Autodesk Inventor part; units mm, degrees
ref_plane "YZ Plane" through (0, 0, 0) normal (1, 0, 0) x (0, 1, 0)
ref_plane "XZ Plane" through (0, 0, 0) normal (0, 1, 0) x (-1, 0, 0)
ref_plane "XY Plane" through (0, 0, 0) normal (0, 0, 1) x (1, 0, 0)
sketch "Sketch1" plane through (0, 0, 0) normal (0, 1, 0) x (-1, 0, 0)
  line L0 (-31, -16.75) -> (31, -16.75)
  line L1 (31, -16.75) -> (31, 16.75)
  line L2 (31, 16.75) -> (-31, 16.75)
  line L3 (-31, 16.75) -> (-31, -16.75)
  line L4 (-31, -16.75) -> (31, 16.75) construction
  line L5 (31, -16.75) -> (-31, 16.75) construction
  point P0 (0, 0)
  dimension "d0" = 33.5
  dimension "d1" = 62
extrude "Extrusion1" add sketch "Sketch1" along normal blind 1.5
fillet "Fillet1" radius 2 4 edges at (31, 0.75, 16.75) (31, 0.75, -16.75) (-31, 0.75, -16.75) (-31, 0.75, 16.75)
sketch "Sketch5" plane through (0, 0, 0) normal (0, -1, 0) x (1, 0, 0)
  line L0 (41, -5) -> (31, -5)
  line L1 (31, -5) -> (31, 5)
  line L2 (31, 5) -> (41, 5)
  line L3 (41, 5) -> (41, -5)
  line L4 (41, -5) -> (31, 5) construction
  line L5 (31, -5) -> (41, 5) construction
  line L6 (31, 14.75) -> (31, -14.75)
  line L7 (-41, -5) -> (-31, -5)
  line L8 (-31, -5) -> (-31, 5)
  line L9 (-31, 5) -> (-41, 5)
  line L10 (-41, 5) -> (-41, -5)
  line L11 (-41, -5) -> (-31, 5) construction
  line L12 (-31, -5) -> (-41, 5) construction
  line L13 (-31, -14.75) -> (-31, 14.75)
  point P0 (0, 0)
  point P1 (36, 0)
  point P2 (36, 0)
  point P3 (-36, 0)
  point P4 (-36, 0)
  dimension "d37" = 10
  dimension "d38" = 10
extrude "Extrusion6" add sketch "Sketch5" against normal up to surface (1.5 mm away)
sketch "Sketch6" plane through (0, 0, 0) normal (0, -1, 0) x (1, 0, 0)
  circle A0 centre (36, 0) radius 1.75
  line L0 (31, 14.75) -> (31, 5)
  circle A1 centre (-36, 0) radius 1.75
  line L1 (-31, 5) -> (-31, 14.75)
  point P0 (0, 0)
  dimension "d41" = 3.5
  dimension "d42" = 5
  dimension "d51" = 5
extrude "Extrusion7" cut sketch "Sketch6" against normal up to surface (1.5 mm away)
fillet "Fillet6" radius 2 8 edges at (31, 0.75, 5) (41, 0.75, 5) (41, 0.75, -5) (31, 0.75, -5) (-31, 0.75, 5) (-41, 0.75, 5) (-41, 0.75, -5) (-31, 0.75, -5)
chamfer "Chamfer1" distance 1.5 angle 45 2 edges at (34.25, 0, 0) (-37.75, 0, 0)
equation "\"d51\" = d42"
properties part number "BatteryPlate"
The listing builds one solid part. Answer for the finished solid, in the listing's coordinates (mm). A direction names the side the tool comes from. Give positions to 0.01 mm unless a question says otherwise; leave off trailing zeros. Order: outer loops, then holes, each group sorted by start corner. A loop starts at its lowest first (then second) coordinate and runs counter-clockwise, first axis right, second up. Notation, with made-up numbers: (70.5, -2) -> (83.5, -2) arc R24 ccw to (83.5, 14) -> close; hole circle Ø5 at (51.25, -36). An arc over 180 degrees is marked (long way). Answer as a JSON object with one key per item and string values. Group by question number.
Item 1: The part is cut by section C-C on y = 0.7. Write down the section's boundary in (x, z), and give its area (3 significant figures).
Item 2: A tool of negligible diameter and unlimited length cuts with its end or side. For faces 1 (the flat face through (36, 1, 5)), 2 (the flat face through (-36, 1, 5)), 3 (the flat face through (36, 1, -5)), 4 (the flat face through (0, 1, -16.75)), 5 (the flat face through (-36, 1, -5)), from which of +Z, -Z, +X, -X, +Y, -Y can it reach the whole face along a straight path? Write none if from no direction.
Item 3: Flat-ended cylindrical pins translate along their axes: pin 1 (0.8 mm diameter, centred on y = 1, z = -11.5, fed in from -X); pin 2 (0.8 mm diameter, centred on x = 36, y = 1, fed in from -Z); pin 3 (0.8 mm diameter, centred on x = -36, y = 0.5, fed in from +Z). Find the tip coordinate at first contact, or state that the pin passes through.
Item 4: The part is cut by section D-D on z = -11.5. Write down the section's boundary in (x, y).
Item 5: The part is cut by section A-A on z = 0. Give the number of separate pieces and of enclosed holes in the cut face, and give its area (3 significant figures).
Item 6: Consider L1, parallel to X at y = 0.75, z = -0.5; L2, parallel to X at y = 0.7, z = -1; L3, parallel to X at y = 0.7, z = 13. Determine where each line is inside the solid, lowest interval first. Write a range as from..to.
Result set:
{
 "1": {"outline": "(-41, -3) arc R2 ccw to (-39, -5) -> (-33, -5) arc R2 cw to (-31, -7) -> (-31, -14.75) arc R2 ccw to (-29, -16.75) -> (29, -16.75) arc R2 ccw to (31, -14.75) -> (31, -7) arc R2 cw to (33, -5) -> (39, -5) arc R2 ccw to (41, -3) -> (41, 3) arc R2 ccw to (39, 5) -> (33, 5) arc R2 cw to (31, 7) -> (31, 14.75) arc R2 ccw to (29, 16.75) -> (-29, 16.75) arc R2 ccw to (-31, 14.75) -> (-31, 7) arc R2 cw to (-33, 5) -> (-39, 5) arc R2 ccw to (-41, 3) -> close; hole circle Ø5.1 at (-36, 0); hole circle Ø5.1 at (36, 0)", "area": "2,230 mm²"},
 "2": {"face 1": "+Z, +X, +Y, -Y", "face 2": "+Z, -X, +Y, -Y", "face 3": "-Z, +X, +Y, -Y", "face 4": "-Z, +X, -X, +Y, -Y", "face 5": "-Z, -X, +Y, -Y"},
 "3": {"pin 1": "x = -31", "pin 2": "z = -5", "pin 3": "z = 5"},
 "4": {"outline": "(-31, 0) -> (31, 0) -> (31, 1.5) -> (-31, 1.5) -> close"},
 "5": {"separate pieces": "3", "enclosed holes": "0", "area": "108 mm²"},
 "6": {"L1": "-41..-38.45, -33.55..33.55, 38.45..41", "L2": "-41..-38.35, -33.65..33.65, 38.35..41", "L3": "-31..31"}
}
